Source: CAD feature listing. Evaluate the final solid. Frame: model axes, mm. Face numbers are marked on the shaded views. A direction names the side the tool comes from. Round coordinates to 2 decimals unless told otherwise and drop trailing zeros. Write item = value, one per line.
from build123d import *

# Parameters (mm, degrees)
FILLET1_R        = 1.5875
SKETCH2_R        = 10.795
ROUND_BOSS_DEPTH = 3.96875
SKETCH4_R        = 6.35
HOLE_DEPTH       = 6.35
MODULAR_REACH    = 39.644
SKETCH12_R       = 6.35


with BuildPart() as part:
    # Sketch1 → Base-Revolve (revolve)
    with BuildSketch(Plane.XY, mode=Mode.PRIVATE) as base_revolve_sk:
        with BuildLine():
            Line((0, 0), (25.4, 0))
            Line((25.4, 0), (26.9875, 1.5875))
            ThreePointArc((26.9875, 1.5875), (25.010459227, 3.639775536), (24.13, 6.35))
            Line((24.13, 6.35), (17.708087105, 6.35))
            Line((17.708087105, 6.35), (15.875, 3.175))
            Line((15.875, 3.175), (0, 3.175))
            Line((0, 3.175), (0, 0))
        make_face()
    revolve(base_revolve_sk.sketch.rotate(Axis((0, 4.772511252, 0), (0, -1, 0)), 90), axis=Axis((0, 4.772511252, 0), (0, -1, 0)))

    # Fillet1
    fillet1_edges = [part.edges().sort_by_distance(p)[0] for p in [
        (0, 3.175, -15.875),
        (0, 6.35, -17.708087105),
        (0, 6.35, -24.13),
        (0, 1.5875, -26.9875),
    ]]
    fillet(fillet1_edges, radius=FILLET1_R)

    # Sketch2 → Round Boss (add)
    with BuildSketch(Plane(origin=(0, 3.175, 0), x_dir=(-1, 0, 0), z_dir=(0, 1, 0))):
        with Locations(Location((0, 0, 0), (0, 0, 270))):
            Circle(SKETCH2_R)
    extrude(amount=ROUND_BOSS_DEPTH)

    # Sketch4 → hole (cut)
    with BuildSketch(Plane(origin=(0, 0, 0), x_dir=(-1, 0, 0), z_dir=(0, 1, 0))):
        with Locations(Location((0, 0, 0), (0, 0, 90))):
            Circle(SKETCH4_R)
    extrude(amount=HOLE_DEPTH, mode=Mode.SUBTRACT)

    # Sketch12 → Modular (cut, up to next)
    with BuildSketch(Plane(origin=(0, 6.35, 0), x_dir=(-1, 0, 0), z_dir=(0, 1, 0)), mode=Mode.PRIVATE) as modular_sk1:
        with Locations(Location((0, 0, 0), (0, 0, 90))):
            Circle(SKETCH12_R)
    modular_tool1 = extrude(modular_sk1.sketch, amount=MODULAR_REACH, mode=Mode.PRIVATE) & part.part
    add(modular_tool1.solids().sort_by_distance((0, 6.35, 0))[0], mode=Mode.SUBTRACT)


solid = part.part
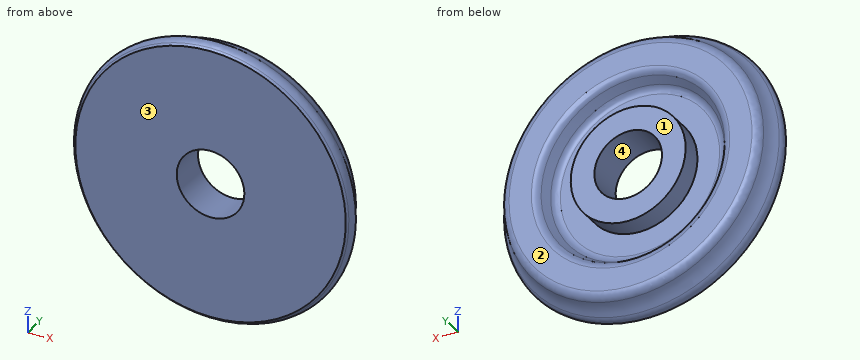
1. Mould query, pull axis X, two halves, no side actions, for the marked faces 3 and 4. Classes: released by +X, released by -X, zero draft, split by the parting line, or undercut.
Evaluation:
face_3 = zero draft
face_4 = undercut
2. Contact query for flat-ended pins moving along their axis: pin 1 Ø15 at (x, z) = (-0.5, -3) entering from +Y; pin 2 Ø4 at (x, y) = (-20, 5) entering from +Z; pin 3 Ø1 at (y, z) = (3.5, -14) entering from +X. Output: stop coordinate, or through.
Evaluation:
pin_1 = 7.14
pin_2 = 16.8
pin_3 = 21.36
3. Line query: probe 1 along Z at (x, y) = (-5, 5.25); probe 2 along X at (y, z) = (3.5, 0) (3 decimals); probe 3 along Z at (x, y) = (-5.5, 6). Output: solid intervals per line, ascending. Write a range as from..to.
Evaluation:
probe_1 = -23.8..-16.32, -9.57..-3.91, 3.91..9.57, 16.32..23.8
probe_2 = -25.097..-15.921, -10.795..-6.35, 6.35..10.795, 15.921..25.097
probe_3 = -23.16..-16.75, -9.29..-3.17, 3.17..9.29, 16.75..23.16
4. Set-up query: the marked faces 1 and 2. Return all of +Z, -Z, +X, -X, +Y, -Y with unobstructed straight access to the full face (end or side cutting, diameter ignored); none if empty.
Evaluation:
face_1 = +Z, -Z, +X, -X, +Y
face_2 = +Y
